Model file for the job. Use its own axes, mm. Face numbers are marked on the shaded views. A direction names the side the tool comes from. Coordinates: 2 decimals unless noted, no trailing zeros. Write each loop counter-clockwise with the first axis right and the second up, starting at its lowest first coordinate (ties: lowest second). Pieces come first, ordered by that corner, then holes.
Q1. Band-saw the part on B-B, the plane z = 0. Write the cut outline in (x, y).
Q2. Which spindle directions (+Z, -Z, +X, -X, +Y, -Y) get a long thin tool onto all of the face, cutting with end or side? Do the marked faces 1, 2, 3, 4 and 5. Say none if no direction does.
Q3. Pin check, flat tips, straight feed: P1, Ø1.2, axis at y = 0, z = 7, coming from the -X side; P2, Ø2, axis at x = 1, z = 8, coming from the -Y side; P3, Ø1.5, axis at x = 3.5, z = 6.5, coming from the -Y side; P4, Ø1, axis at x = 2.5, y = 8.5, coming from the -Z side. Stop position of each tip, or through.
Q4. Pull direction Y, two halves, no side cores. Call the marked faces 6, 7 and 8: released by +Y, released by -Y, zero draft, split by the parting line, or undercut.
Q5. Band-saw the part on A-A, the plane y = 0. Write the cut outline in (x, z), plus the area to 3 significant figures.
Q6. Band-saw the part on D-D, the plane z = 3.75. Write the cut outline in (x, y), plus the area to 3 significant figures.
Q7. Drill centre lines: probe 1 along Y at (x, z) = (1.1, 0); probe 2 along Y at (x, z) = (0.7, 7); probe 3 along Z at (x, y) = (1.3, 7.5). Where is each one in solid material? Low to high.
Q8. Band-saw the part on C-C, the plane x = 4.4. State how many separate pieces and enclosed holes the cut face has, plus the area to 3 significant figures.
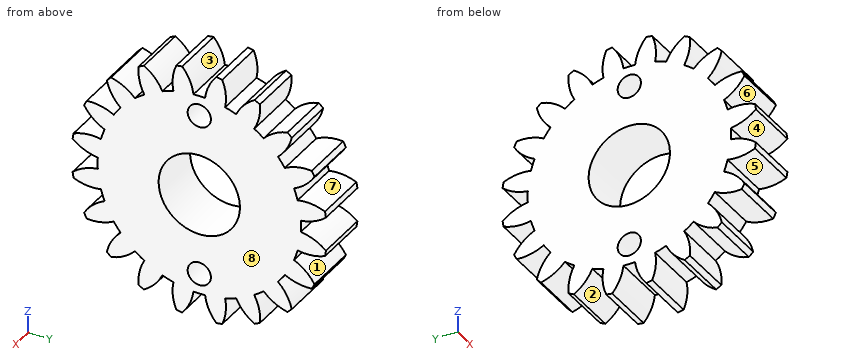
from build123d import *

# Parameters (mm, degrees)
BASPROSKE_W        = 4.7
BASPROSKE_H        = 11
TOOTHCUT_DEPTH     = 17.250846132
TEETHCUTS_COUNT    = 20
TEETHCUTS_ANGLE    = 342
BORSKE_R           = 3.5
BORE_DEPTH         = 50.0000508
SKETCH1_R          = 1
CUT_EXTRUDE1_DEPTH = 17.118244485


with BuildPart() as part:
    # BasProSke → Base-Revolve (revolve)
    with BuildSketch(Plane(origin=(0, 0, 0), x_dir=(1, 0, 0), z_dir=(0, 1, 0)), mode=Mode.PRIVATE) as base_revolve_sk:
        with Locations((2.35, 5.5)):
            Rectangle(BASPROSKE_W, BASPROSKE_H)
    revolve(base_revolve_sk.sketch.rotate(Axis((-10, 0, 0), (1, 0, 0)), 180), axis=Axis((-10, 0, 0), (1, 0, 0)))

    # TooCutSke → ToothCut (cut, through all)
    with BuildSketch(Plane(origin=(0, 0, 0), x_dir=(0, 0, -1), z_dir=(1, 0, 0))):
        with BuildLine():
            ThreePointArc((0.499924007, 8.734705318), (0, 8.749), (-0.499924007, 8.734705318))
            ThreePointArc((-0.499924007, 8.734705318), (-0.824302243, 9.905497836), (-1.485192705, 10.924909509))
            ThreePointArc((-1.485192705, 10.924909509), (0, 11.0254), (1.485192705, 10.924909509))
            ThreePointArc((1.485192705, 10.924909509), (0.824302243, 9.905497836), (0.499924007, 8.734705318))
        make_face()
    toothcut = extrude(amount=TOOTHCUT_DEPTH, mode=Mode.SUBTRACT)

    # TeethCuts: ToothCut ×20 about axis
    teethcuts_axis = Axis((-10, 0, 0), (1, 0, 0))
    for i in range(1, TEETHCUTS_COUNT):
        add(toothcut.rotate(teethcuts_axis, i * TEETHCUTS_ANGLE / (TEETHCUTS_COUNT - 1)), mode=Mode.SUBTRACT)

    # BorSke → Bore (cut, symmetric)
    with BuildSketch(Plane(origin=(0, 0, 0), x_dir=(0, 0, -1), z_dir=(1, 0, 0))):
        with Locations(Location((0, 0, 0), (0, 0, 180))):
            Circle(BORSKE_R)
    extrude(amount=BORE_DEPTH, both=True, mode=Mode.SUBTRACT)

    # Sketch1 → Cut-Extrude1 (cut, through all)
    with BuildSketch(Plane(origin=(4.7, 0, 0), x_dir=(0, 0, -1), z_dir=(1, 0, 0))):
        with Locations((-7, 0)):
            Circle(SKETCH1_R)
        with Locations((7, 0)):
            Circle(SKETCH1_R)
    extrude(amount=-CUT_EXTRUDE1_DEPTH, mode=Mode.SUBTRACT)


solid = part.part
Answer sheet:
1. outline: (0, -8.75) - (4.7, -8.75) - (4.7, -3.5) - (0, -3.5) - close; (0, 3.5) - (4.7, 3.5) - (4.7, 8.75) - (0, 8.75) - close
2. face 1: +X, -X, +Y
2. face 2: -Z, +X, -X
2. face 3: +Z, +X, -X
2. face 4: +X, -X, -Y
2. face 5: +X, -X
3. P1: passes through
3. P2: stops at y = -7.96
3. P3: stops at y = -7.86
3. P4: stops at z = -5.23
4. face 6: released by -Y
4. face 7: undercut
4. face 8: zero draft
5. outline: (0, -8.75) - (4.7, -8.75) - (4.7, -8) - (0, -8) - close; (0, -6) - (4.7, -6) - (4.7, -3.5) - (0, -3.5) - close; (0, 3.5) - (4.7, 3.5) - (4.7, 6) - (0, 6) - close; (0, 8) - (4.7, 8) - (4.7, 8.75) - (0, 8.75) - close
5. area: 30.5 mm2
6. outline: (0, -9.06) - (4.7, -9.06) - (4.7, 9.06) - (0, 9.06) - close
6. area: 85.1 mm2
7. probe 1: y = -8.75 to -3.5, 3.5 to 8.75
7. probe 2: y = -7.78 to -5.77, -5.25 to -1, 1 to 5.25, 5.77 to 7.78
7. probe 3: z = -7.94 to -6.44, -4.8 to 4.8, 6.44 to 7.94
8. separate pieces: 1
8. enclosed holes: 3
8. area: 258 mm2
